from build123d import *

# Parameters (mm, degrees)
PAD009_DEPTH    = 20
SKETCH023_R     = 3
POCKET008_DEPTH = 44.001
SKETCH024_R     = 3
POCKET009_DEPTH = 5
SKETCH026_W     = 44
SKETCH026_H     = 4
PAD011_DEPTH    = 20
SKETCH027_W     = 20
SKETCH027_H     = 10
SKETCH027_W_2   = 14
SKETCH027_H_2   = 4
PAD012_DEPTH    = 20
SKETCH028_R     = 1.4
POCKET010_DEPTH = 3


with BuildPart() as part:
    # Sketch021 → Pad009 (new body)
    with BuildSketch(Plane.XY):
        with BuildLine():
            Line((0, -44), (0, 0))
            Line((0, 0), (20, 0))
            Line((20, 0), (20, -5))
            Line((20, -5), (7, -5))
            ThreePointArc((7, -5), (4.87868, -5.87868), (4, -8))
            Line((4, -8), (4, -44))
            Line((4, -44), (0, -44))
        make_face()
    extrude(amount=PAD009_DEPTH)

    # Sketch023 → Pocket008 (cut, through all)
    with BuildSketch(Plane.XZ):
        with Locations((14, 15)):
            Circle(SKETCH023_R)
    extrude(amount=POCKET008_DEPTH, mode=Mode.SUBTRACT)

    # Sketch024 → Pocket009 (cut)
    with BuildSketch(Plane.YZ):
        with Locations((-38, 9)):
            Circle(SKETCH024_R)
    extrude(amount=POCKET009_DEPTH, mode=Mode.SUBTRACT)

    # Sketch026 → Pad011 (join)
    with BuildSketch(Plane.YZ):
        with Locations((-22, 22)):
            Rectangle(SKETCH026_W, SKETCH026_H)
    extrude(amount=PAD011_DEPTH)

    # Sketch027 → Pad012 (join)
    with BuildSketch(Plane.YZ):
        with Locations((-34, 29)):
            Rectangle(SKETCH027_W, SKETCH027_H)
        with Locations((-34, 29)):
            Rectangle(SKETCH027_W_2, SKETCH027_H_2, mode=Mode.SUBTRACT)
    extrude(amount=PAD012_DEPTH)

    # Sketch028 → Pocket010 (cut)
    with BuildSketch(Plane.XY.offset(34)):
        with Locations((10, -34)):
            Circle(SKETCH028_R)
    extrude(amount=-POCKET010_DEPTH, mode=Mode.SUBTRACT)


solid = part.part
Geometry check sheet. Reference: the model listing, model coordinates, mm. A direction names the side the tool comes from. Round coordinates to 2 decimals unless told otherwise and drop trailing zeros. Loops run counter-clockwise (first coordinate to the right, second up) from the corner with the lowest first, then second, coordinate; pieces in that order, holes last. Notation, with made-up numbers: (76, -8.5) - (121, -8.5) arc R18 cw to (121, -3.5) - close; hole circle Ø9 at (78, 41). An arc over 180 degrees is marked (long way). One line per question, with ' | ' between items. Start each with the question number.
1. Cross-section at A-A on x = 14. Record the cut outline in (y, z).
2. Draft check along X on faces 5 (the face through (10, -12, 24)), 6 (the face through (11.6, -2.5, 13.2)), 7 (the face through (20, -22, 21)). Enter one of: released by +X, released by -X, zero draft, split by the parting line, or undercut.
3. Tool access check on faces 1 (the face through (9.82, -32.61, 32.52)), 2 (the face through (10, -34, 27)), 3 (the face through (4.9, -5.86, 9.86)), 4 (the face through (10, -24, 29)). Record the directions out of +Z, -Z, +X, -X, +Y, -Y that give a thin tool (end or side, any length) a straight path to the whole face; none if there is none.
4. Scan lines: line 1 (Z direction, x = 7.5, y = -40); line 2 (Y direction, x = 10, z = 32.55); line 3 (Y direction, x = 15.5, z = 29.5). Record each from-to range of solid material in increasing order. Write a range as [from, to].
5. Cross-section at B-B on y = -38. Record the cut outline in (x, z), then the cut area to 3 significant figures.
6. Cross-section at D-D on y = -30. Record the cut outline in (x, z).
7. Depth check by flat-ended pin: pin 1 (2 mm diameter, centred on x = 9, y = -23, fed in from -Z); pin 2 (2 mm diameter, centred on x = 13, z = 29, fed in from +Y); pin 3 (16 mm diameter, centred on y = -32, z = 7, fed in from +X). Enter the tip coordinate at first touch or a pass-through.
8. Cross-section at C-C on z = 9. Record the cut outline in (x, y).
Taken from the geometry:
1) outline: (-44, 20) - (-5, 20) - (-5, 18) - (0, 18) - (0, 24) - (-24, 24) - (-24, 34) - (-44, 34) - close; (-5, 0) - (0, 0) - (0, 12) - (-5, 12) - close; hole (-41, 27) - (-27, 27) - (-27, 31) - (-41, 31) - close
2) face 5: zero draft | face 6: undercut | face 7: released by +X
3) face 1: +Z | face 2: +X, -X | face 3: -Z, +X, -Y | face 4: +Z, +X, -X, +Y
4) line 1: [20, 27], [31, 34] | line 2: [-44, -35.4], [-32.6, -24] | line 3: [-44, -41], [-27, -24]
5) outline: (0, 0) - (4, 0) - (4, 6) - (0, 6) - close; (0, 12) - (4, 12) - (4, 20) - (20, 20) - (20, 27) - (0, 27) - close; (0, 31) - (20, 31) - (20, 34) - (0, 34) - close | area: 256 mm²
6) outline: (0, 0) - (4, 0) - (4, 20) - (20, 20) - (20, 27) - (0, 27) - close; (0, 31) - (20, 31) - (20, 34) - (0, 34) - close
7) pin 1: z = 20 | pin 2: y = -24 | pin 3: x = 4
8) outline: (0, -44) - (4, -44) - (4, -41) - (0, -41) - close; (0, -35) - (4, -35) - (4, -8) arc R3 cw to (7, -5) - (20, -5) - (20, 0) - (0, 0) - close
